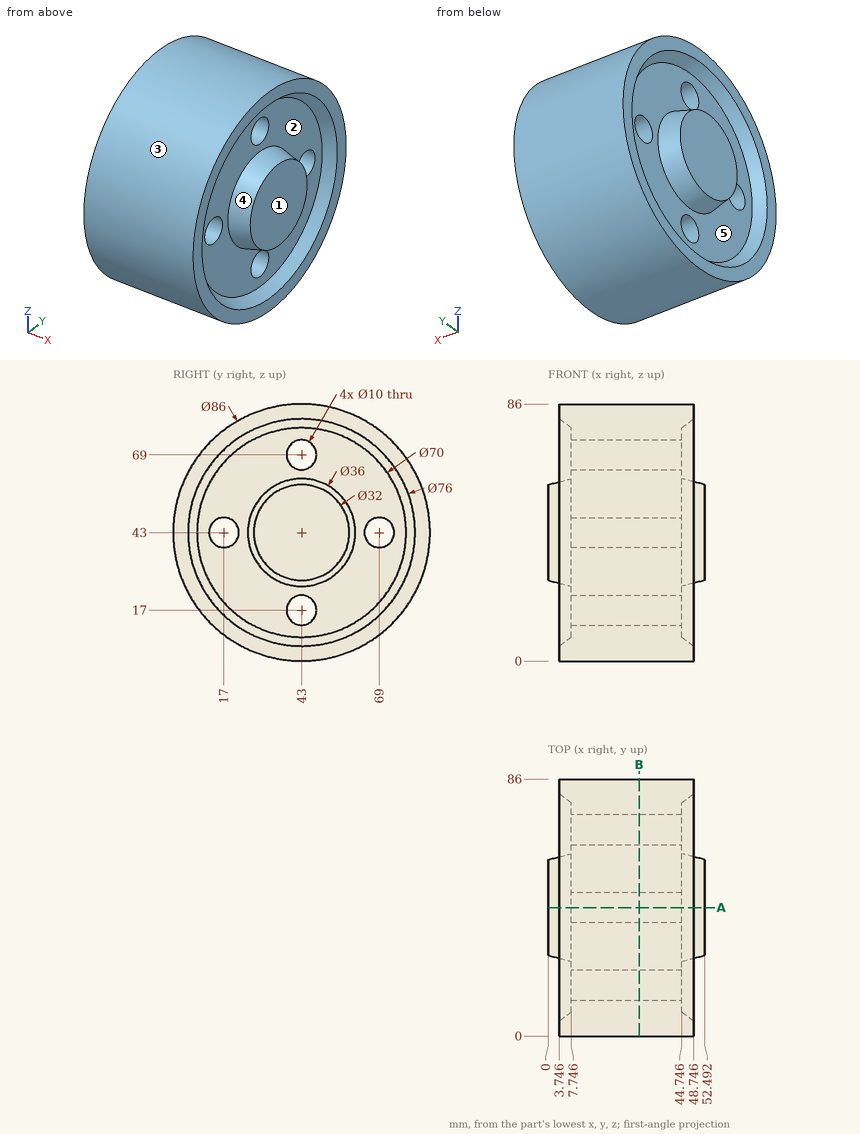
Job drawing, mm, ordinate dimensions from the low corner. One solid piece. A direction names the side the tool comes from. Coordinates: 2 decimals unless noted, no trailing zeros. Order: outer loops, then holes, each group sorted by start corner. A loop starts at its lowest first (then second) coordinate and runs counter-clockwise, first axis right, second up. Notation, with made-up numbers: (55, 86) -> (82, 86) arc R24 cw to (82, 96) -> close; hole circle Ø7 at (8, 22.25). An arc over 180 degrees is marked (long way). Return JSON: item names as keys, results as strings. Group by question number.
Item 1: Wall check: line 1 along Z through (x, y) = (17, 43); line 2 along Y through (x, z) = (42.5, 46) (1 decimal); line 3 along Z through (x, y) = (46, 36.5). Give the ranges that are in metal, low to high. Write a range as [from, to].
Item 2: Flat gauge pins, fed straight in: P1, Ø1.5, axis at x = 27.5, z = 50, coming from the +Y side; P2, Ø11.5, axis at y = 17, z = 43, coming from the +X side; P3, Ø1, axis at x = 42.5, y = 71, coming from the +Z side. Where does each tip first touch, or does it go through?
Item 3: Tool access for the marked faces 4 and 5: list every direction of +Z, -Z, +X, -X, +Y, -Y with a clear straight run to the whole face (end or side of a thin tool).
Item 4: Saw through at A-A on y = 43. Write the cut outline in (x, z).
Item 5: Pull direction Z, two halves, no side cores. Call the marked faces 1, 2 and 3: pulls with the +Z half, pulls with the -Z half, needs draft (parallel to the pull), parting line crosses it, or undercut.
Item 6: Saw through at B-B on x = 30.5. Write the cut outline in (y, z).
Values found:
{
 "1": {"line 1": "z = [0, 12], [22, 64], [74, 86]", "line 2": "y = [0.1, 13], [21, 65], [73, 85.9]", "line 3": "z = [0.49, 7.65], [26.56, 59.44], [78.35, 85.51]"},
 "2": {"P1": "stops at y = 85.54", "P2": "stops at x = 44.75", "P3": "stops at z = 76.06"},
 "3": {"face 4": "+X", "face 5": "-X"},
 "4": {"outline": "(0, 27) -> (7.75, 25) -> (7.75, 22) -> (44.75, 22) -> (44.75, 25) -> (52.49, 27) -> (52.49, 59) -> (44.75, 61) -> (44.75, 64) -> (7.75, 64) -> (7.75, 61) -> (0, 59) -> close; (3.75, 0) -> (48.75, 0) -> (48.75, 5) -> (44.75, 8) -> (44.75, 12) -> (7.75, 12) -> (7.75, 8) -> (3.75, 5) -> close; (3.75, 81) -> (7.75, 78) -> (7.75, 74) -> (44.75, 74) -> (44.75, 78) -> (48.75, 81) -> (48.75, 86) -> (3.75, 86) -> close"},
 "5": {"face 1": "needs draft", "face 2": "undercut", "face 3": "parting line crosses it"},
 "6": {"outline": "circle Ø86 at (43, 43); hole circle Ø10 at (17, 43); hole circle Ø10 at (43, 17); hole circle Ø10 at (43, 69); hole circle Ø10 at (69, 43)"}
}
